Input: dimensioned drawing with shaded views. Units: mm. Origin: part minimum x, y, z. Give positions to 0.01 mm unless a question says otherwise; leave off trailing zeros. Order: outer loops, then holes, each group sorted by start corner. A loop starts at its lowest first (then second) coordinate and runs counter-clockwise, first axis right, second up. Notation, with made-up numbers: (63, 50) - (115, 50) arc R22 ccw to (115, 87) - close; hole circle Ø11 at (76, 34.5). An arc over 180 degrees is marked (long way). Use a Markdown table: item, result.
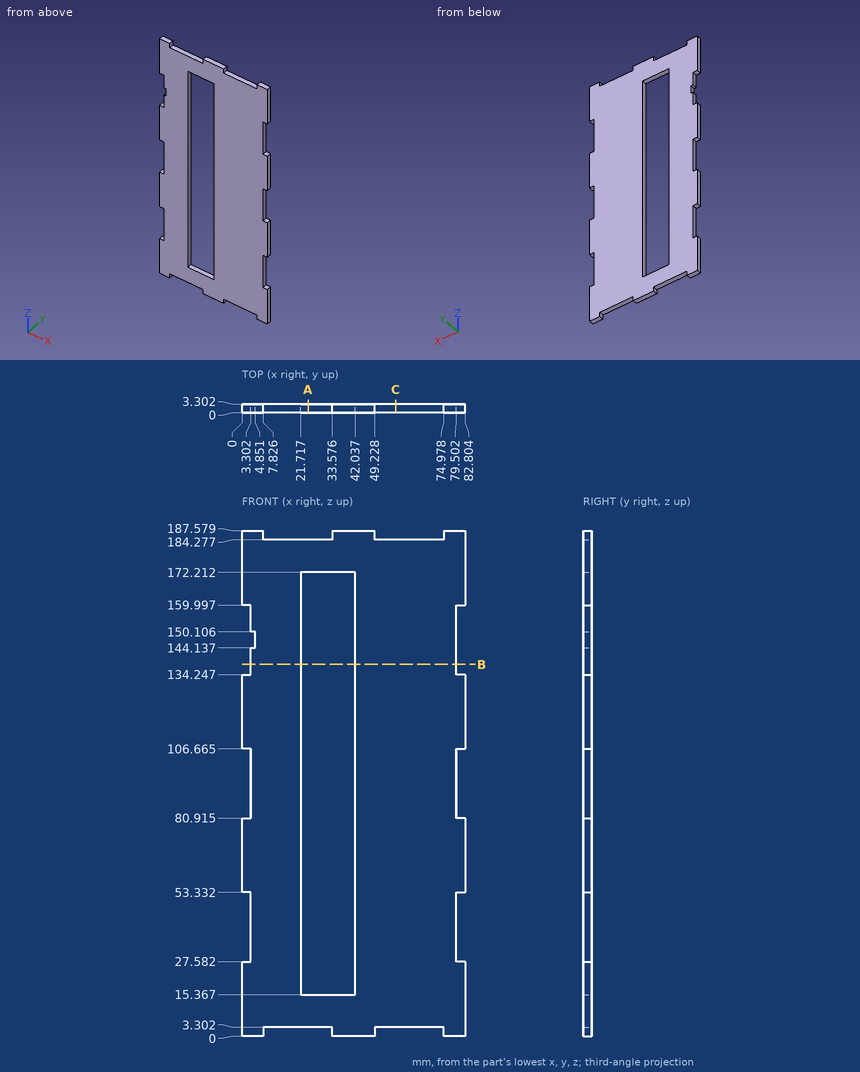
1. Material intervals for line 1 along Z through (x, y) = (34, 3.05); line 2 along Z through (x, y) = (22, 0.55); line 3 along X through (y, z) = (1.7, 101.5), sorted ascending.
Response:
| item | result |
|---|---|
| line 1 | z = 0 to 15.37, 172.21 to 187.58 |
| line 2 | z = 3.3 to 15.37, 172.21 to 184.28 |
| line 3 | x = 3.3 to 21.72, 42.04 to 79.5 |
2. Section query B-B (z = 138). Return loops of the section in (x, y).
Response:
| item | result |
|---|---|
| outline | (3.3, 0) - (21.72, 0) - (21.72, 3.3) - (3.3, 3.3) - close; (42.04, 0) - (79.5, 0) - (79.5, 3.3) - (42.04, 3.3) - close |
3. Section query C-C (x = 57). Return loops of the section in (y, z).
Response:
| item | result |
|---|---|
| outline | (0, 3.3) - (3.3, 3.3) - (3.3, 184.28) - (0, 184.28) - close |
4. Pin query (flat end, axial travel): pin 1 (1 mm diameter, centred on y = 1, z = 186, fed in from -X); pin 2 (1 mm diameter, centred on x = 63.5, y = 1.5, fed in from +Z); pin 3 (1 mm diameter, centred on y = 2, z = 96.5, fed in from -X); pin 4 (1 mm diameter, centred on y = 2, z = 44.5, fed in from +X). Return the tip coordinate at first contact, or that it passes through.
Response:
| item | result |
|---|---|
| pin 1 | stops at x = 0 |
| pin 2 | stops at z = 184.28 |
| pin 3 | stops at x = 3.3 |
| pin 4 | stops at x = 79.5 |
5. Section query A-A (x = 24.5). Return loops of the section in (y, z).
Response:
| item | result |
|---|---|
| outline | (0, 3.3) - (3.3, 3.3) - (3.3, 15.37) - (0, 15.37) - close; (0, 172.21) - (3.3, 172.21) - (3.3, 184.28) - (0, 184.28) - close |
